Check sheet for the modelled part. Datum: model origin and axes. Units: mm. A direction names the side the tool comes from. Give positions to 0.01 mm unless a question says otherwise; leave off trailing zeros. Write each loop counter-clockwise with the first axis right and the second up, starting at its lowest first coordinate (ties: lowest second). Pieces come first, ordered by that corner, then holes. Notation, with made-up numbers: M 10.25,20.5 L 68.25,20.5 A20 cw 68.25,28.5 Z; hole C 56,52 d2. An arc over 180 degrees is marked long. Write item = value, one per line. Start each with the question number.
1) Sectioned sample at D-D, the plane y = 8. Record the cut outline in (x, z), then the cut area to 3 significant figures.
2) Draft check along X on faces 1 (the face through (8.87, 29.44, 1.5)), 2 (the face through (-37.23, -31.27, 7.4)), 3 (the face through (52.01, 29.37, 6.04)), 4 (the face through (46.696, -26.363, 7.395)). Enter one of: pulls with the +X half, pulls with the -X half, needs draft (parallel to the pull), parting line crosses it, or undercut.
3) Sectioned sample at A-A, the plane x = 36.5. Record the cut outline in (y, z), then the cut area to 3 significant figures.
4) Scan lines: L1, parallel to Y at x = 47.5, z = 6.5; L2, parallel to Y at x = 22, z = 10.25; L3, parallel to Y at x = 47, z = 12.75. Record each from-to range of solid material in increasing order.
5) Sectioned sample at B-B, the plane z = 7. Record the cut outline in (x, y), then the cut area to 3 significant figures.
6) Sectioned sample at C-C, the plane x = -27.5. Record the cut outline in (y, z), then the cut area to 3 significant figures.
7) Gauge pin test, flat ends, axial feed: pin 1 (1.5 mm diameter, centred on x = 12, z = 8, fed in from +Y); pin 2 (1.5 mm diameter, centred on y = 7.5, z = 4.5, fed in from -X). Record the tip position at first contact, or that the pin passes through.
8) Set-up check for faces 5 (the face through (3.96, 29.44, 13.5)), 6 (the face through (-46.15, -4.619, 13.496)), 7 (the face through (6, 30.871, 7)): record each of +Z, -Z, +X, -X, +Y, -Y from which the full face is reachable in a straight line by a thin tool's end or side.
from build123d import *

# Parameters (mm, degrees)
F0_R         = 3.586786404
F0_R_2       = 3.7582992631
F0_R_3       = 3.6865102679
F1_DEPTH     = 15
F2_T1_DEPTH  = 126.0138504207
F2_T3_DEPTH  = 22.5
F2_T5_DEPTH  = 74.126155749
F2_S9_W      = 5
F2_S9_H      = 5
F2_T10_DEPTH = 5
F2_T16_DEPTH = 97.9066217834
F2_S17_R     = 6.9574459714
F2_T18_DEPTH = 51
F2_T22_DEPTH = 82.9931766736
F2_S23_R     = 6.9574459714
F2_T24_DEPTH = 43
F2_T28_ANGLE = 359.64
F2_T34_ANGLE = 359.64
F2_T40_ANGLE = 359.64
F2_T46_DEPTH = 115.4066217834
F2_S47_R     = 6.9574459714
F2_T48_DEPTH = 59
F2_T53_ANGLE = 359.64
F2_T58_DEPTH = 97.9066217834
F2_S59_R     = 6.9574459714
F2_T60_DEPTH = 51
F2_T66_ANGLE = 359.64
F2_T71_DEPTH = 82.9931766736
F2_S72_R     = 6.9574459714
F2_T73_DEPTH = 43


# Not quite as in the source:
# - a fillet or chamfer that OpenCascade refuses, or shapes differently, is made with other operations: its cross-section is extruded or revolved along the edge and cut away or added


with BuildPart() as f1:
    # F0 (on Top) → F1 (new body)
    with BuildSketch(Plane.XY):
        with BuildLine():
            Line((-47.5761555135, 22.2377919602), (-47.5761555135, 30.8707710356))
            Line((-47.5761555135, 30.8707710356), (-36.9689268762, 30.8707710356))
            ThreePointArc((-36.9689268762, 30.8707710356), (-47.4740962985, 32.9453643179), (-47.5761555135, 22.2377919602))
        make_face()
        with BuildLine():
            Line((-36.9689268762, 30.8707710356), (-47.5761555135, 30.8707710356))
            Line((-47.5761555135, 30.8707710356), (-47.5761555135, 22.2377919602))
            ThreePointArc((-47.5761555135, 22.2377919602), (-40.1548216165, 21.2376644422), (-36.1248620528, 27.5492314249))
            ThreePointArc((-36.1248620528, 27.5492314249), (-36.3391791701, 29.2627855393), (-36.9689268762, 30.8707710356))
        make_face()
        with BuildLine():
            Line((53.4376949072, 30.8707710356), (-36.9689268762, 30.8707710356))
            ThreePointArc((-36.9689268762, 30.8707710356), (-36.3391791701, 29.2627855393), (-36.1248620528, 27.5492314249))
            ThreePointArc((-36.1248620528, 27.5492314249), (-40.1548216165, 21.2376644422), (-47.5761555135, 22.2377919602))
            Line((-47.5761555135, 22.2377919602), (-47.5761555135, -35.7553847134))
            Line((-47.5761555135, -35.7553847134), (53.4376949072, -35.7553847134))
            Line((53.4376949072, -35.7553847134), (53.4376949072, 30.8707710356))
        make_face()
        with Locations((-40.5423082411, -29.8938471824)):
            Circle(F0_R, mode=Mode.SUBTRACT)
        with Locations((47.1853874624, -30.089231208)):
            Circle(F0_R_2, mode=Mode.SUBTRACT)
        with Locations((38.5884605348, 26.1815395206)):
            Circle(F0_R_3, mode=Mode.SUBTRACT)
    extrude(amount=F1_DEPTH)

    # F2: fillet of radius 5 on 7 edges, made by hand

    # F2_s2 → F2_t1 (cut)
    with BuildSketch(Plane.YZ.offset(-60.0761555135)):
        with BuildLine():
            ThreePointArc((-35.7553847134, 10), (-34.2909186193, 13.5355339059), (-30.7553847134, 15))
            Line((-30.7553847134, 15), (-35.7553847134, 15))
            Line((-35.7553847134, 15), (-35.7553847134, 10))
        make_face()
    extrude(amount=F2_T1_DEPTH, mode=Mode.SUBTRACT)

    # F2_s4 → F2_t3 (cut)
    with BuildSketch(Plane.XY.offset(-12.5)):
        with BuildLine():
            ThreePointArc((53.4376949072, 25.8707710356), (51.9732288131, 29.4063049415), (48.4376949072, 30.8707710356))
            Line((48.4376949072, 30.8707710356), (53.4376949072, 30.8707710356))
            Line((53.4376949072, 30.8707710356), (53.4376949072, 25.8707710356))
        make_face()
    extrude(amount=F2_T3_DEPTH, mode=Mode.SUBTRACT)

    # F2_s6 → F2_t5 (cut)
    with BuildSketch(Plane.XZ.offset(-25.8707710356)):
        with BuildLine():
            ThreePointArc((53.4376949072, 10), (51.9732288131, 13.5355339059), (48.4376949072, 15))
            Line((48.4376949072, 15), (53.4376949072, 15))
            Line((53.4376949072, 15), (53.4376949072, 10))
        make_face()
    extrude(amount=F2_T5_DEPTH, mode=Mode.SUBTRACT)


with BuildPart() as f2_tool8:
    # F2_s9 → F2_t10 (new body)
    with BuildSketch(Plane.XY.offset(10)):
        with Locations((50.9376949072, 28.3707710356)):
            Rectangle(F2_S9_W, F2_S9_H)
    extrude(amount=F2_T10_DEPTH)

    # F2_s11 → F2_t12 (revolve, cut)
    with BuildSketch(Plane(origin=(48.4376949072, 25.8707710356, 10), x_dir=(-0.7071067812, -0.7071067812, 0), z_dir=(-0.7071067812, 0.7071067812, 0))):
        with BuildLine():
            ThreePointArc((0, -5), (5, 0), (0, 5))
            Line((0, 5), (0, -5))
        make_face()
    revolve(axis=Axis((48.4376949072, 25.8707710356, 10), (0, 0, 1)), mode=Mode.SUBTRACT)


with BuildPart() as f1_1:
    add(f1.part)

    # F2_t7: cut F2_tool8
    add(f2_tool8.part, mode=Mode.SUBTRACT)


with BuildPart() as f2_tool14:
    # F2_s15 → F2_t16 (new body)
    with BuildSketch(Plane.YZ.offset(48.4376949072)):
        with BuildLine():
            ThreePointArc((30.8707710356, 10), (29.4063049415, 13.5355339059), (25.8707710356, 15))
            Line((25.8707710356, 15), (30.8707710356, 15))
            Line((30.8707710356, 15), (30.8707710356, 10))
        make_face()
    extrude(amount=-F2_T16_DEPTH)

    # F2_s17 → F2_t18 (cut, symmetric)
    with BuildSketch(Plane.XY.offset(12.5)):
        with Locations((-43.0823080242, 27.5492314249)):
            Circle(F2_S17_R)
    extrude(amount=F2_T18_DEPTH, both=True, mode=Mode.SUBTRACT)


with BuildPart() as f1_2:
    add(f1_1.part)

    # F2_t13: cut F2_tool14
    add(f2_tool14.part, mode=Mode.SUBTRACT)


with BuildPart() as f2_tool20:
    # F2_s21 → F2_t22 (new body)
    with BuildSketch(Plane.XZ.offset(-34.7377919602)):
        with BuildLine():
            ThreePointArc((-47.5761555135, 10), (-46.1116894195, 13.5355339059), (-42.5761555135, 15))
            Line((-42.5761555135, 15), (-47.5761555135, 15))
            Line((-47.5761555135, 15), (-47.5761555135, 10))
        make_face()
    extrude(amount=F2_T22_DEPTH)

    # F2_s23 → F2_t24 (cut, symmetric)
    with BuildSketch(Plane.XY.offset(12.5)):
        with Locations((-43.0823080242, 27.5492314249)):
            Circle(F2_S23_R)
    extrude(amount=F2_T24_DEPTH, both=True, mode=Mode.SUBTRACT)


with BuildPart() as f1_3:
    add(f1_2.part)

    # F2_t19: cut F2_tool20
    add(f2_tool20.part, mode=Mode.SUBTRACT)


with BuildPart() as f2_tool26:
    # F2_s27 → F2_t28 (revolve)
    with BuildSketch(Plane(origin=(-12.2782997509, -10.0573142374, 0), x_dir=(0, 0, 1), z_dir=(-0.77360415, -0.6336691716, 0))):
        with BuildLine():
            ThreePointArc((10, 41.6546842262), (13.5355339059, 43.1191503203), (15, 46.6546842262))
            Line((15, 46.6546842262), (15, 41.6546842262))
            Line((15, 41.6546842262), (10, 41.6546842262))
        make_face()
    revolve(axis=Axis((-43.0823080242, 27.5492314249, 15), (0, 0, 1)), revolution_arc=F2_T28_ANGLE)

    split(bisect_by=Plane.XZ.offset(-30.8707710356), keep=Keep.TOP)

    split(bisect_by=Plane.YZ.offset(-47.5761555135), keep=Keep.BOTTOM)


with BuildPart() as f1_4:
    add(f1_3.part)

    # F2_t25: cut F2_tool26
    add(f2_tool26.part, mode=Mode.SUBTRACT)


with BuildPart() as f2_tool32:
    # F2_s33 → F2_t34 (revolve)
    with BuildSketch(Plane(origin=(-12.2782997509, -10.0573142374, 0), x_dir=(0, 0, 1), z_dir=(-0.77360415, -0.6336691716, 0))):
        with BuildLine():
            ThreePointArc((10, 41.6546842262), (13.5355339059, 43.1191503203), (15, 46.6546842262))
            Line((15, 46.6546842262), (15, 41.6546842262))
            Line((15, 41.6546842262), (10, 41.6546842262))
        make_face()
    revolve(axis=Axis((-43.0823080242, 27.5492314249, 15), (0, 0, 1)), revolution_arc=F2_T34_ANGLE)

    split(bisect_by=Plane.XZ.offset(-30.8707710356), keep=Keep.BOTTOM)

    split(bisect_by=Plane.YZ.offset(-47.5761555135), keep=Keep.TOP)


with BuildPart() as f1_5:
    add(f1_4.part)

    # F2_t31: cut F2_tool32
    add(f2_tool32.part, mode=Mode.SUBTRACT)


with BuildPart() as f2_tool38:
    # F2_s39 → F2_t40 (revolve)
    with BuildSketch(Plane(origin=(-12.2782997509, -10.0573142374, 0), x_dir=(0, 0, 1), z_dir=(-0.77360415, -0.6336691716, 0))):
        with BuildLine():
            ThreePointArc((10, 41.6546842262), (13.5355339059, 43.1191503203), (15, 46.6546842262))
            Line((15, 46.6546842262), (15, 41.6546842262))
            Line((15, 41.6546842262), (10, 41.6546842262))
        make_face()
    revolve(axis=Axis((-43.0823080242, 27.5492314249, 15), (0, 0, 1)), revolution_arc=F2_T40_ANGLE)

    split(bisect_by=Plane.XZ.offset(-30.8707710356), keep=Keep.BOTTOM)

    split(bisect_by=Plane.YZ.offset(-47.5761555135), keep=Keep.BOTTOM)


with BuildPart() as f1_6:
    add(f1_5.part)

    # F2_t37: cut F2_tool38
    add(f2_tool38.part, mode=Mode.SUBTRACT)


with BuildPart() as f2_tool44:
    # F2_s45 → F2_t46 (new body)
    with BuildSketch(Plane.YZ.offset(65.9376949072)):
        with BuildLine():
            ThreePointArc((30.8707710356, 5), (29.4063049415, 1.4644660941), (25.8707710356, 0))
            Line((25.8707710356, 0), (30.8707710356, 0))
            Line((30.8707710356, 0), (30.8707710356, 5))
        make_face()
    extrude(amount=-F2_T46_DEPTH)

    # F2_s47 → F2_t48 (cut, symmetric)
    with BuildSketch(Plane.XY.offset(2.5)):
        with Locations((-43.0823080242, 27.5492314249)):
            Circle(F2_S47_R)
    extrude(amount=F2_T48_DEPTH, both=True, mode=Mode.SUBTRACT)


with BuildPart() as f1_7:
    add(f1_6.part)

    # F2_t43: cut F2_tool44
    add(f2_tool44.part, mode=Mode.SUBTRACT)


with BuildPart() as f2_tool51:
    # F2_s52 → F2_t53 (revolve)
    with BuildSketch(Plane(origin=(-12.2782997509, -10.0573142374, 0), x_dir=(0, 0, 1), z_dir=(-0.77360415, -0.6336691716, 0))):
        with BuildLine():
            ThreePointArc((10, 41.6546842262), (13.5355339059, 43.1191503203), (15, 46.6546842262))
            Line((15, 46.6546842262), (15, 41.6546842262))
            Line((15, 41.6546842262), (10, 41.6546842262))
        make_face()
    revolve(axis=Axis((-43.0823080242, 27.5492314249, 15), (0, 0, 1)), revolution_arc=F2_T53_ANGLE)

    split(bisect_by=Plane.XZ.offset(-30.8707710356), keep=Keep.TOP)

    split(bisect_by=Plane.YZ.offset(-47.5761555135), keep=Keep.TOP)


with BuildPart() as f2_tool56:
    # F2_s57 → F2_t58 (new body)
    with BuildSketch(Plane.YZ.offset(48.4376949072)):
        with BuildLine():
            ThreePointArc((30.8707710356, 10), (29.4063049415, 13.5355339059), (25.8707710356, 15))
            Line((25.8707710356, 15), (30.8707710356, 15))
            Line((30.8707710356, 15), (30.8707710356, 10))
        make_face()
    extrude(amount=-F2_T58_DEPTH)

    # F2_s59 → F2_t60 (intersect, symmetric)
    with BuildSketch(Plane.XY.offset(12.5)):
        with Locations((-43.0823080242, 27.5492314249)):
            Circle(F2_S59_R)
    extrude(amount=F2_T60_DEPTH, both=True, mode=Mode.INTERSECT)


with BuildPart() as f2_tool51_1:
    add(f2_tool51.part)

    # F2_t61: intersect F2_tool56
    add(f2_tool56.part, mode=Mode.INTERSECT)


with BuildPart() as f1_8:
    add(f1_7.part)

    # F2_t49: cut F2_tool51
    add(f2_tool51_1.part, mode=Mode.SUBTRACT)


with BuildPart() as f2_tool64:
    # F2_s65 → F2_t66 (revolve)
    with BuildSketch(Plane(origin=(-12.2782997509, -10.0573142374, 0), x_dir=(0, 0, 1), z_dir=(-0.77360415, -0.6336691716, 0))):
        with BuildLine():
            ThreePointArc((10, 41.6546842262), (13.5355339059, 43.1191503203), (15, 46.6546842262))
            Line((15, 46.6546842262), (15, 41.6546842262))
            Line((15, 41.6546842262), (10, 41.6546842262))
        make_face()
    revolve(axis=Axis((-43.0823080242, 27.5492314249, 15), (0, 0, 1)), revolution_arc=F2_T66_ANGLE)

    split(bisect_by=Plane.XZ.offset(-30.8707710356), keep=Keep.TOP)

    split(bisect_by=Plane.YZ.offset(-47.5761555135), keep=Keep.TOP)


with BuildPart() as f2_tool69:
    # F2_s70 → F2_t71 (new body)
    with BuildSketch(Plane.XZ.offset(-34.7377919602)):
        with BuildLine():
            ThreePointArc((-47.5761555135, 10), (-46.1116894195, 13.5355339059), (-42.5761555135, 15))
            Line((-42.5761555135, 15), (-47.5761555135, 15))
            Line((-47.5761555135, 15), (-47.5761555135, 10))
        make_face()
    extrude(amount=F2_T71_DEPTH)

    # F2_s72 → F2_t73 (intersect, symmetric)
    with BuildSketch(Plane.XY.offset(12.5)):
        with Locations((-43.0823080242, 27.5492314249)):
            Circle(F2_S72_R)
    extrude(amount=F2_T73_DEPTH, both=True, mode=Mode.INTERSECT)


with BuildPart() as f2_tool64_1:
    add(f2_tool64.part)

    # F2_t74: intersect F2_tool69
    add(f2_tool69.part, mode=Mode.INTERSECT)


with BuildPart() as f1_9:
    add(f1_8.part)

    # F2_t62: cut F2_tool64
    add(f2_tool64_1.part, mode=Mode.SUBTRACT)


solid = f1_9.part
Data:
q1.outline = M -47.58,0 L 53.44,0 L 53.44,10 A5 ccw 48.44,15 L -42.58,15 A5 ccw -47.58,10 Z
q1.area = 1,500 mm2
q2.face_1 = needs draft
q2.face_2 = undercut
q2.face_3 = pulls with the +X half
q2.face_4 = undercut
q3.outline = M -35.76,0 L 23.14,0 L 23.14,15 L -30.76,15 A5 ccw -35.76,10 Z; M 29.22,1.29 A5 ccw 30.87,5 L 30.87,10 A5 ccw 29.22,13.71 Z
q3.area = 895 mm2
q4.L1 = -35.76 to -33.83, -26.34 to 30.87
q4.L2 = -35.75 to 30.86
q4.L3 = -34.93 to -33.84, -26.34 to 30.05
q5.outline = M -47.58,-35.76 L 53.44,-35.76 L 53.44,25.87 A5 ccw 48.44,30.87 L -36.97,30.87 A6.96 ccw long -47.58,22.24 Z; hole C -40.54,-29.89 d7.17; hole C 38.59,26.18 d7.37; hole C 47.19,-30.09 d7.52
q5.area = 6,650 mm2
q6.outline = M -35.76,0 L 25.87,0 A5 ccw 30.87,5 L 30.87,10 A5 ccw 25.87,15 L -30.76,15 A5 ccw -35.76,10 Z
q6.area = 983 mm2
q7.pin_1 = 30.87
q7.pin_2 = -47.58
q8.face_5 = +Z, +X, +Y
q8.face_6 = +Z, -X, -Y
q8.face_7 = +Z, -Z, +X, +Y
